Autodesk Inventor part; units mm, degrees
ref_plane "YZ Plane" through (0, 0, 0) normal (1, 0, 0) x (0, 1, 0)
ref_plane "XZ Plane" through (0, 0, 0) normal (0, 1, 0) x (-1, 0, 0)
ref_plane "XY Plane" through (0, 0, 0) normal (0, 0, 1) x (1, 0, 0)
sketch "Sketch1" plane through (0, 0, 0) normal (0, 1, 0) x (-1, 0, 0)
  line L0 (0, 0) -> (40.5, 0)
  line L1 (40.5, 0) -> (40.5, -20.33)
  line L2 (40.5, -20.33) -> (0, -20.33)
  line L3 (0, -20.33) -> (0, 0)
  dimension "d0" = 20.33
  dimension "d1" = 40.5
extrude "Extrusion1" add sketch "Sketch1" along normal blind 27.77
sketch "Sketch2" plane through (0, 27.77, 0) normal (0, 1, 0) x (1, 0, 0)
  line L0 (8, 0) -> (-48.5, 0)
  line L1 (-48.5, 0) -> (-48.5, 20.33)
  line L2 (-48.5, 20.33) -> (8, 20.33)
  line L3 (8, 20.33) -> (8, 0)
  line L4 (0, 20.33) -> (-40.5, 20.33)
  line L5 (-40.5, 20.33) -> (-40.5, 0)
  line L6 (-40.5, 0) -> (0, 0)
  line L7 (0, 0) -> (0, 20.33)
  point P0 (-40.5, 20.33)
  dimension "d4" = 0
  dimension "d6" = 8
  dimension "d7" = 0
  dimension "d41" = 8
extrude "Extrusion2" add sketch "Sketch2" along normal blind 2.59
sketch "Sketch3" plane through (0, 30.36, 0) normal (0, 1, 0) x (1, 0, 0)
  circle A0 centre (-44.5, 5) radius 2.5
  circle A1 centre (-44.5, 15.33) radius 2.5
  line L0 (-48.5, 0) -> (8, 0)
  line L1 (8, 20.33) -> (-48.5, 20.33)
  line L2 (-48.5, 20.33) -> (-48.5, 0)
  point P0 (0, 0)
  dimension "d10" = 5
  dimension "d11" = 5
  dimension "d12" = 5
  dimension "d14" = 5
  dimension "d15" = 4
  dimension "d16" = 4
extrude "Extrusion3" cut sketch "Sketch3" against normal blind 3.5
ref_plane "Work Plane1" through (-20.25, 27.77, 0) normal (1, 0, 0) x (0, 0, -1)
mirror "Mirror1" about plane through (-20.25, 27.77, 0) normal (1, 0, 0) of "Extrusion3"
sketch "Sketch4" plane through (0, 30.36, 0) normal (0, 1, 0) x (1, 0, 0)
  line L0 (0, 0) -> (-40.5, 0)
  line L1 (-40.5, 0) -> (-40.5, 20.33)
  line L2 (-40.5, 20.33) -> (0, 20.33)
  line L3 (0, 20.33) -> (0, 0)
extrude "Extrusion4" add sketch "Sketch4" along normal blind 10
sketch "Sketch5" plane through (0, 40.36, 0) normal (0, 1, 0) x (1, 0, 0)
  circle A0 centre (-11, 10) radius 2.83
  line L0 (0, 0) -> (0, 20.33)
  line L1 (-40.5, 0) -> (0, 0)
  line L2 (-40.5, 20.33) -> (-40.5, 0)
  dimension "d22" = 10
  dimension "d23" = 5.66
  dimension "d42" = 11
extrude "Extrusion5" add sketch "Sketch5" along normal blind 4
sketch "Sketch6" plane through (0, 0, 0) normal (1, 0, 0) x (0, 0, -1)
  line L0 (6.75, 3) -> (13.25, 3)
  line L1 (13.25, 3) -> (13.25, 6.5)
  line L2 (13.25, 6.5) -> (6.75, 6.5)
  line L3 (6.75, 6.5) -> (6.75, 3)
  line L4 (0, 0) -> (20.33, 0)
  line L5 (0, 0) -> (0, 27.77)
  dimension "d26" = 3
  dimension "d27" = 6.5
  dimension "d28" = 3.5
  dimension "d29" = 6.75
extrude "Extrusion6" add sketch "Sketch6" along normal blind 6
sketch "Sketch7" plane through (6, 0, 0) normal (1, 0, 0) x (0, 0, -1)
  circle A0 centre (11.75, 4.75) radius 1.5
  circle A1 centre (8.25, 4.75) radius 1.5
  line L0 (6.75, 6.5) -> (6.75, 3)
  line L1 (13.25, 3) -> (13.25, 6.5)
  line L2 (6.75, 3) -> (13.25, 3)
  point P0 (0, 0)
  dimension "d32" = 3
  dimension "d33" = 3
  dimension "d34" = 1.5
  dimension "d35" = 1.5
  dimension "d36" = 1.75
  dimension "d37" = 1.75
extrude "Extrusion7" add sketch "Sketch7" along normal blind 30
equation "\"d16\" = d15"
equation "\"d33\" = d32"
equation "\"d37\" = d36"
properties part number "motor_25kg"
Geometry check sheet. Reference: the model listing, model coordinates, mm. A direction names the side the tool comes from. Give positions to 0.01 mm unless a question says otherwise; leave off trailing zeros. Write each loop counter-clockwise with the first axis right and the second up, starting at its lowest first coordinate (ties: lowest second). Pieces come first, ordered by that corner, then holes. Notation, with made-up numbers: M -18,-22 L 39,-22 A23 ccw 39,-3 Z; hole C 44.25,58.25 d1. An arc over 180 degrees is marked long. Answer as CSV lines item,"result". Start each with the question number.
Q1. Release check for a two-part mould opening along Y. For faces 1 (the face through (1.615, 29.083, -4.249)), 2 (the face through (3, 6.5, -10)), 3 (the face through (3, 3, -10)), 4 (the face through (4, 30.36, -10)) record: pulls with the +Y half, pulls with the -Y half, needs draft (parallel to the pull), parting line crosses it, or undercut.
Q2. Section check D-D, the plane x = 24.5. Record the cut outline in (y, z).
Q3. Go/stop test with flat-tipped pins: pin 1 (6 mm diameter, centred on y = 37.5, z = -7.5, fed in from +X); pin 2 (4 mm diameter, centred on x = 4, z = -5, fed in from +Y); pin 3 (8 mm diameter, centred on x = 9.5, y = 24.5, fed in from -Z); pin 4 (10 mm diameter, centred on x = -24.5, z = -5.5, fed in from +Y). Record where each tip stops, or that it passes through.
Q4. Tool access check on faces 5 (the face through (-45, 30.36, -10)), 6 (the face through (4.54, 29.08, -17.77)), 7 (the face through (8, 29, -10)), 8 (the face through (4, 27.77, -10)). Record the directions out of +Z, -Z, +X, -X, +Y, -Y that give a thin tool (end or side, any length) a straight path to the whole face; none if there is none.
Q5. Section check B-B, the plane z = -5. Record the cut outline in (x, y).
Q6. Material ranges on L1, parallel to X at y = 29.35, z = -15.33; L2, parallel to Z at x = -44.5, y = 29.5; L3, parallel to X at y = 26, z = -8, recorded low to high.
Q7. Section check C-C, the plane z = -11.5. Record the cut outline in (x, y).
Q8. Section check A-A, the plane x = -44.5. Record the cut outline in (y, z), then the cut area to 3 significant figures.
Geometry says:
1,face 1,"needs draft"
1,face 2,"undercut"
1,face 3,"pulls with the -Y half"
1,face 4,"pulls with the +Y half"
2,outline,"C 4.75,-11.75 d3; C 4.75,-8.25 d3"
3,pin 1,"x = 0"
3,pin 2,"y = 6.5"
3,pin 3,"z = -20.33"
3,pin 4,"y = 40.36"
4,face 5,"+Z, -Z, -X, +Y"
4,face 6,"+Y"
4,face 7,"+Z, -Z, +X, +Y"
4,face 8,"+Z, -Z, +X"
5,outline,"M -48.5,27.77 L -47,27.77 L -47,30.36 L -48.5,30.36 Z; M -42,27.77 L -40.5,27.77 L -40.5,0 L 0,0 L 0,27.77 L 1.5,27.77 L 1.5,30.36 L 0,30.36 L 0,40.36 L -40.5,40.36 L -40.5,30.36 L -42,30.36 Z; M 6.5,27.77 L 8,27.77 L 8,30.36 L 6.5,30.36 Z"
6,L1,"-48.5 to -47, -42 to 1.5, 6.5 to 8"
6,L2,"-20.33 to -17.83, -12.83 to -7.5, -2.5 to 0"
6,L3,"-40.5 to 0"
7,outline,"M -48.5,27.77 L -40.5,27.77 L -40.5,0 L 0,0 L 0,3 L 6,3 L 6,3.27 L 36,3.27 L 36,6.23 L 6,6.23 L 6,6.5 L 0,6.5 L 0,27.77 L 8,27.77 L 8,30.36 L 0,30.36 L 0,40.36 L -8.6,40.36 L -8.6,44.36 L -13.4,44.36 L -13.4,40.36 L -40.5,40.36 L -40.5,30.36 L -48.5,30.36 Z"
8,outline,"M 27.77,-20.33 L 30.36,-20.33 L 30.36,-17.83 L 27.77,-17.83 Z; M 27.77,-12.83 L 30.36,-12.83 L 30.36,-7.5 L 27.77,-7.5 Z; M 27.77,-2.5 L 30.36,-2.5 L 30.36,0 L 27.77,0 Z"
8,area,"26.8 mm^2"
